from build123d import *

# Parameters (mm, degrees)
SKETCH1_W                                            = 200
SKETCH1_H                                            = 200
BOSS_EXTRUDE1_DEPTH                                  = 19.05
SKETCH2_W                                            = 200
SKETCH2_H                                            = 3.05
CUT_EXTRUDE1_DEPTH                                   = 225.416805298
SKETCH3_R                                            = 90.5
CUT_EXTRUDE2_DEPTH                                   = 6
M12_TAPPED_HOLE1_D                                   = 10.2
M12_TAPPED_HOLE1_DEPTH                               = 32.75
M12_TAPPED_HOLE1_TIP                                 = 3.064389157
SKETCH6_R                                            = 48.41875
CUT_EXTRUDE3_DEPTH                                   = 144.791515744
FILLET1_R                                            = 0.79375
CBORE_FOR_M10_HEX_SOCKET_HEAD_CAP_SCREW1_D           = 11
CBORE_FOR_M10_HEX_SOCKET_HEAD_CAP_SCREW1_CBORE_D     = 18
CBORE_FOR_M10_HEX_SOCKET_HEAD_CAP_SCREW1_CBORE_DEPTH = 17


with BuildPart() as part:
    # Sketch1 → Boss-Extrude1 (new, symmetric)
    with BuildSketch(Plane(origin=(0, 0, 0), x_dir=(1, 0, 0), z_dir=(0, 1, 0))):
        Rectangle(SKETCH1_W, SKETCH1_H)
    extrude(amount=BOSS_EXTRUDE1_DEPTH, both=True)

    # Sketch2 → Cut-Extrude1 (cut, through all)
    with BuildSketch(Plane.XY.offset(100)):
        with Locations((0, 17.525)):
            Rectangle(SKETCH2_W, SKETCH2_H)
        with Locations((0, -17.525)):
            Rectangle(SKETCH2_W, SKETCH2_H)
    extrude(amount=-CUT_EXTRUDE1_DEPTH, mode=Mode.SUBTRACT)

    # Sketch3 → Cut-Extrude2 (cut)
    with BuildSketch(Plane(origin=(0, 16, 0), x_dir=(1, 0, 0), z_dir=(0, 1, 0))):
        with Locations(Location((0, 0, 0), (0, 0, 270))):
            Circle(SKETCH3_R)
    extrude(amount=-CUT_EXTRUDE2_DEPTH, mode=Mode.SUBTRACT)

    # M12 Tapped Hole1
    with Locations(Plane(origin=(0, 16, 0), x_dir=(1, 0, 0), z_dir=(0, 1, 0))):
        with Locations((-76.013978978, 76.013978978), (76.013978978, 76.013978978), (76.013978978, -76.013978978), (-76.013978978, -76.013978978)):
            Hole(M12_TAPPED_HOLE1_D / 2, depth=M12_TAPPED_HOLE1_DEPTH)
            with Locations((0, 0, -(M12_TAPPED_HOLE1_DEPTH + M12_TAPPED_HOLE1_TIP / 2))):  # 118° drill point
                Cone(0, M12_TAPPED_HOLE1_D / 2, M12_TAPPED_HOLE1_TIP, mode=Mode.SUBTRACT)

    # Sketch6 → Cut-Extrude3 (cut, through all)
    with BuildSketch(Plane(origin=(0, 10, 0), x_dir=(1, 0, 0), z_dir=(0, 1, 0))):
        with Locations(Location((0, 0, 0), (0, 0, 270))):
            Circle(SKETCH6_R)
    extrude(amount=-CUT_EXTRUDE3_DEPTH, mode=Mode.SUBTRACT)

    # Fillet1
    fillet1_edges = [part.edges().sort_by_distance(p)[0] for p in [
        (0, 10, -90.5),
    ]]
    fillet(fillet1_edges, radius=FILLET1_R)

    # CBORE for M10 Hex Socket Head Cap Screw1 (through all)
    with Locations(Plane(origin=(0, 16, 0), x_dir=(1, 0, 0), z_dir=(0, 1, 0))):
        with Locations((-67.5, -50), (-67.5, 0), (-67.5, 50), (67.5, 50), (67.5, 0), (67.5, -50)):
            CounterBoreHole(CBORE_FOR_M10_HEX_SOCKET_HEAD_CAP_SCREW1_D / 2, CBORE_FOR_M10_HEX_SOCKET_HEAD_CAP_SCREW1_CBORE_D / 2, CBORE_FOR_M10_HEX_SOCKET_HEAD_CAP_SCREW1_CBORE_DEPTH)


solid = part.part
Input: part model. Units: mm. Frame: model coordinates. A direction names the side the tool comes from. Give positions to 0.01 mm unless a question says otherwise; leave off trailing zeros. Order: outer loops, then holes, each group sorted by start corner. A loop starts at its lowest first (then second) coordinate and runs counter-clockwise, first axis right, second up.
Q1. Set-up query: faces 1 (the cylindrical face through (73, -9, 50)), 2 (the flat face through (63, -1, 54)). Return all of +Z, -Z, +X, -X, +Y, -Y with unobstructed straight access to the full face (end or side cutting, diameter ignored); none if empty.
Checked values:
face 1: +Y, -Y
face 2: +Y
Q2. Ray query, probe 1 along X at (y, z) = (0.5, 76); probe 2 along X at (y, z) = (5, -50); probe 3 along Z at (x, y) = (67.5, -5.5). Return the intervals inside material, ascending.
Checked values:
probe 1: x = -100 to -81.11, -70.91 to 70.91, 81.11 to 100
probe 2: x = -100 to -76.5, -58.5 to 58.5, 76.5 to 100
probe 3: z = -100 to -55.5, -44.5 to -5.5, 5.5 to 44.5, 55.5 to 100
Q3. Section A-A on x = 0. Output: boundary loops of the cut face in (y, z), and give its area (3 significant figures).
Checked values:
outline: (-16, -100) - (16, -100) - (16, -90.5) - (10.79, -90.5) arc R0.79 cw to (10, -89.71) - (10, -48.42) - (-16, -48.42) - close; (-16, 48.42) - (10, 48.42) - (10, 89.71) arc R0.79 cw to (10.79, 90.5) - (16, 90.5) - (16, 100) - (-16, 100) - close
area: 2,800 mm2
Q4. Section B-B on y = 7.5. State how many separate pieces and enclosed holes the cut face has, and give its area (3 significant figures).
Checked values:
separate pieces: 1
enclosed holes: 11
area: 30,800 mm2
Q5. Draft query along Z for faces 3 (the flat face through (-90, 16, 24)), 4 (the cylindrical face through (-58.916, 4.577, -2.703)), 5 (the flat face through (-1, 0, -100)), 6 (the flat face through (-1, 0, 100)). Return one class per face: +Z half, -Z half, draft (parallel to the pull), parting line (faces both ways), or undercut.
Checked values:
face 3: draft
face 4: undercut
face 5: -Z half
face 6: +Z half
Q6. Contact query for flat-ended pins moving along their axis: pin 1 Ø9 at (x, z) = (-76.01, 76.01) entering from +Y; pin 2 Ø14.5 at (x, z) = (69, -1.5) entering from +Y. Output: stop coordinate, or through.
Checked values:
pin 1: passes through
pin 2: stops at y = 10
